Geometry check sheet. Reference: drawing and pictorial views, mm from the part's lowest x, y, z. A direction names the side the tool comes from. Round coordinates to 2 decimals unless told otherwise and drop trailing zeros. Loops run counter-clockwise (first coordinate to the right, second up) from the corner with the lowest first, then second, coordinate; pieces in that order, holes last. Notation, with made-up numbers: (16.5, 52.25) - (65.5, 52.25) arc R30 ccw to (65.5, 75.25) - close; hole circle Ø10 at (61, -27.5). An arc over 180 degrees is marked (long way). Answer as CSV lines item,"result". Start each with the question number.
1) Depth check by flat-ended pin: P1, Ø10, axis at x = 57, z = 72, coming from the +Y side. Enter the tip coordinate at first touch or a pass-through.
2) Cross-section at A-A on z = 12. Record the boundary of the cut face in (x, y), and give its area (3 significant figures).
3) Access from +Z, -Z, +X, -X, +Y, -Y to the whole of each face (thin tool, end or side, straight path). Record for the marked faces 4 and 5.
4) Cross-section at C-C on x = 120. Record the boundary of the cut face in (y, z), and give its area (3 significant figures).
5) Thickness scan on line 1 along Z through (x, y) = (101, 40); line 2 along X through (y, z) = (130, 123.5); line 3 along Y through (x, z) = (86, 61). Record the ranges inside material, lowest first.
6) Draft check along Z on the marked faces 1, 2 and 3. Enter one of: released by +Z, released by -Z, zero draft, split by the parting line, or undercut.
7) Cross-section at B-B on y = 28.5. Record the boundary of the cut face in (x, z).
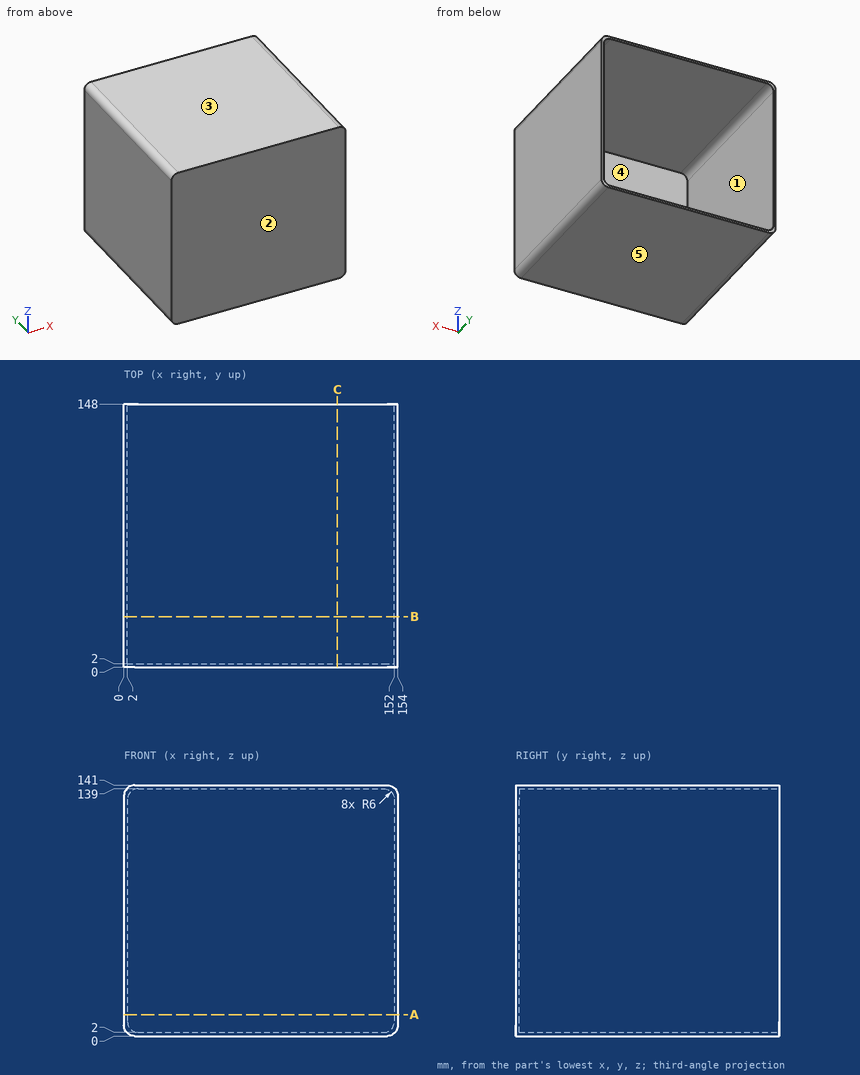
Answer block:
1,P1,"stops at y = 2"
2,outline,"(0, 0) - (154, 0) - (154, 148) - (152, 148) - (152, 2) - (2, 2) - (2, 148) - (0, 148) - close"
2,area,"892 mm^2"
3,face 4,"+Y"
3,face 5,"-Z, +X, -X, +Y, -Y"
4,outline,"(0, 0) - (148, 0) - (148, 2) - (2, 2) - (2, 139) - (148, 139) - (148, 141) - (0, 141) - close"
4,area,"866 mm^2"
5,line 1,"z = 0 to 2, 139 to 141"
5,line 2,"x = 0 to 2, 152 to 154"
5,line 3,"y = 0 to 2"
6,face 1,"undercut"
6,face 2,"zero draft"
6,face 3,"released by +Z"
7,outline,"(0, 6) arc R6 ccw to (6, 0) - (148, 0) arc R6 ccw to (154, 6) - (154, 135) arc R6 ccw to (148, 141) - (6, 141) arc R6 ccw to (0, 135) - close; hole (2, 8) arc R6 ccw to (8, 2) - (146, 2) arc R6 ccw to (152, 8) - (152, 133) arc R6 ccw to (146, 139) - (8, 139) arc R6 ccw to (2, 133) - close"
